For this review, take the finished solid that the model builds, in its own axes (mm). Face numbers are marked on the shaded views. A direction names the side the tool comes from. Coordinates: 2 decimals unless noted, no trailing zeros. Loops run counter-clockwise (first coordinate to the right, second up) from the corner with the lowest first, then second, coordinate; pieces in that order, holes last. Notation, with made-up numbers: (5, 10.5) -> (35, 10.5) arc R32 cw to (35, 38.5) -> close; hole circle Ø6 at (-0.75, 39). An arc over 180 degrees is marked (long way). Use a Markdown table: item, result.
Autodesk Inventor part; units mm, degrees
ref_plane "YZ Plane" through (0, 0, 0) normal (1, 0, 0) x (0, 1, 0)
ref_plane "XZ Plane" through (0, 0, 0) normal (0, 1, 0) x (-1, 0, 0)
ref_plane "XY Plane" through (0, 0, 0) normal (0, 0, 1) x (1, 0, 0)
sketch "Sketch1" plane through (0, 0, 0) normal (1, 0, 0) x (0, 1, 0)
  line L0 (0, 7.5) -> (0, 15)
  line L1 (0, 15) -> (5, 15)
  line L2 (5, 15) -> (5, 2)
  line L3 (5, 2) -> (9, 2)
  line L4 (9, 2) -> (9, 4)
  line L5 (9, 4) -> (10, 4)
  line L6 (10, 4) -> (10, 0.65)
  line L7 (10, 0.65) -> (3, 0.65)
  line L8 (3, 0.65) -> (3, 7.5)
  line L9 (3, 7.5) -> (0, 7.5)
  line L10 (-2, 0) -> (12, 0)
  point P0 (0, 0)
  dimension "d0" = 7.5
  dimension "d1" = 0.65
  dimension "d2" = 4
  dimension "d3" = 2
  dimension "d4" = 15
  dimension "d5" = 5
  dimension "d6" = 4
  dimension "d7" = 1
  dimension "d34" = 3
revolve "Revolution1" add sketch "Sketch1" angle 360 about axis through (0, -10, 0) along (0, 1, 0)
sketch "Sketch2" plane through (0, 0, 0) normal (0, -1, 0) x (1, 0, 0)
  point P0 (0, 0)
  point P1 (0, -12)
  dimension "d10" = 12
hole "Hole1" at (0, 0, -12) direction (0, 1, 0) diameter 3 end through all
pattern_circular "Circular Pattern1" count 3 over 360 about axis through (0, 2.5, 0) along (0, 1, 0) of "Hole1"
sketch "Sketch3" plane through (0, 0, 0) normal (0, -1, 0) x (1, 0, 0)
  circle A0 centre (0, 0) radius 12 construction
  circle A1 centre (0, -12) radius 1.5
  point P0 (-10.3923, -6)
  dimension "d21" = 24
  dimension "d22" = 60
hole "Hole2" at (-10.3923, 0, -6) direction (0, 1, 0) diameter 2.459 end through all
pattern_circular "Circular Pattern2" count 3 over 360 about axis through (0, 2.5, 0) along (0, 1, 0) of "Hole2"
sketch "Sketch4" plane through (0, 3, 0) normal (0, -1, 0) x (1, 0, 0)
  point P0 (0, 0)
  point P1 (0, 0)
hole "Hole3" at (0, 3, 0) direction (0, 1, 0) diameter 3.2 depth 5 tip angle 118
properties part number "RodHolder-2023-1" material "Copper"
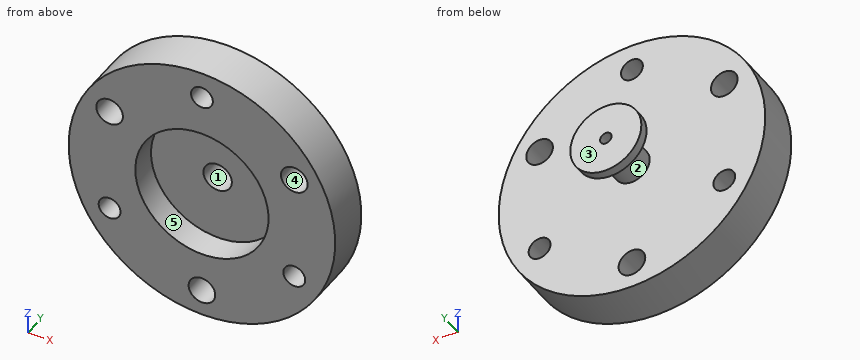
(1) For pin 1 Ø12 at (x, z) = (0, 0) entering from -Y; pin 2 Ø3 at (x, z) = (-10.39, -6) entering from +Y; pin 3 Ø2.5 at (x, z) = (10.39, 6) entering from +Y; pin 4 Ø3 at (y, z) = (4, -4.5) entering from +X, all flat-tipped, find the tip position at first contact; note any pin that passes through.
Found:
| item | result |
|---|---|
| pin 1 | stops at y = 3 |
| pin 2 | stops at y = 5 |
| pin 3 | passes through |
| pin 4 | stops at x = 14.7 |
(2) For the marked faces 4 and 5, list the 3-axis set-ups (+Z, -Z, +X, -X, +Y, -Y) from which the entire face can be reached by the end or side of a thin tool; tool diameter is ignored.
Found:
| item | result |
|---|---|
| face 4 | +Y, -Y |
| face 5 | -Y |
(3) For line 1 along X through (y, z) = (8.9, 0); line 2 along Z through (x, y) = (-9.5, 4.25); line 3 along Z through (x, y) = (-10.5, 4), list the stretches that pass through material, from the lowest coordinate up.
Found:
| item | result |
|---|---|
| line 1 | x = -2 to -0.65, 0.65 to 2 |
| line 2 | z = -11.61 to -6.85, -5.15 to 4.79, 7.21 to 11.61 |
| line 3 | z = -10.71 to -7.22, -4.78 to 4.5, 7.5 to 10.71 |
(4) Take a section at A-A on z = 0. Write out the cut boundary in (x, y).
Found:
| item | result |
|---|---|
| outline | (-15, 0) -> (-7.5, 0) -> (-7.5, 3) -> (-1.6, 3) -> (-1.6, 8) -> (-0.65, 8.57) -> (-0.65, 10) -> (-4, 10) -> (-4, 9) -> (-2, 9) -> (-2, 5) -> (-15, 5) -> close; (0.65, 8.57) -> (1.6, 8) -> (1.6, 3) -> (7.5, 3) -> (7.5, 0) -> (15, 0) -> (15, 5) -> (2, 5) -> (2, 9) -> (4, 9) -> (4, 10) -> (0.65, 10) -> close |
(5) Take a section at C-C on x = -2.5. Write out the cut boundary in (y, z), plus the area to 3 significant figures.
Found:
| item | result |
|---|---|
| outline | (0, -14.79) -> (5, -14.79) -> (5, 14.79) -> (0, 14.79) -> (0, 7.07) -> (3, 7.07) -> (3, -7.07) -> (0, -7.07) -> close; (9, -3.12) -> (10, -3.12) -> (10, 3.12) -> (9, 3.12) -> close |
| area | 112 mm^2 |
(6) Mouldability with a two-part tool opening along X and no side actions: class the marked faces 1, 2 and 3 as pulls with the +X half, pulls with the -X half, needs draft (parallel to the pull), parting line crosses it, or undercut.
Found:
| item | result |
|---|---|
| face 1 | undercut |
| face 2 | parting line crosses it |
| face 3 | needs draft |
(7) Take a section at B-B on z = -5.75. Write out the cut boundary in (x, y).
Found:
| item | result |
|---|---|
| outline | (-13.85, 0) -> (-11.6, 0) -> (-11.6, 5) -> (-13.85, 5) -> close; (-9.19, 0) -> (-4.82, 0) -> (-4.82, 3) -> (4.82, 3) -> (4.82, 0) -> (9.19, 0) -> (9.19, 5) -> (-9.19, 5) -> close; (11.6, 0) -> (13.85, 0) -> (13.85, 5) -> (11.6, 5) -> close |
